Geometry check sheet. Reference: drawing and pictorial views, mm from the part's lowest x, y, z. A direction names the side the tool comes from. Round coordinates to 2 decimals unless told otherwise and drop trailing zeros. Write each loop counter-clockwise with the first axis right and the second up, starting at its lowest first coordinate (ties: lowest second). Pieces come first, ordered by that corner, then holes. Notation, with made-up numbers: M 13.25,54 L 64.25,54 A6 ccw 64.25,59 Z; hole C -18,-22.5 d11. An arc over 180 degrees is marked long. Answer in a Markdown table with one row per item.
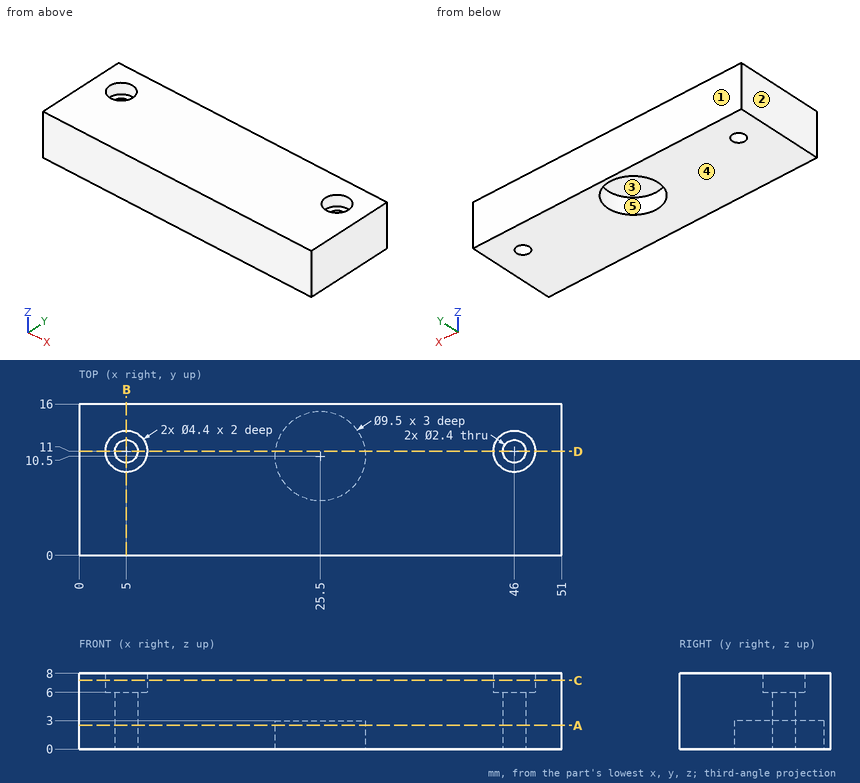
1. Section check A-A, the plane z = 2.5. Record the cut outline in (x, y), and give its area (3 significant figures).
Found:
| item | result |
|---|---|
| outline | M 0,0 L 51,0 L 51,16 L 0,16 Z; hole C 5,11 d2.4; hole C 25.5,10.5 d9.5; hole C 46,11 d2.4 |
| area | 736 mm2 |
2. Scan lines: L1, parallel to X at y = 11, z = 4.25; L2, parallel to Y at x = 46, z = 3.05; L3, parallel to X at y = 11, z = 7.35. Record each from-to range of solid material in increasing order.
Found:
| item | result |
|---|---|
| L1 | x = 0 to 3.8, 6.2 to 44.8, 47.2 to 51 |
| L2 | y = 0 to 9.8, 12.2 to 16 |
| L3 | x = 0 to 2.8, 7.2 to 43.8, 48.2 to 51 |
3. Access from +Z, -Z, +X, -X, +Y, -Y to the whole of each face (thin tool, end or side, straight path). Record for the marked faces 4 and 5.
Found:
| item | result |
|---|---|
| face 4 | -Z, +X, -X, +Y, -Y |
| face 5 | -Z |
4. Section check C-C, the plane z = 7.25. Record the cut outline in (x, y), and give its area (3 significant figures).
Found:
| item | result |
|---|---|
| outline | M 0,0 L 51,0 L 51,16 L 0,16 Z; hole C 5,11 d4.4; hole C 46,11 d4.4 |
| area | 786 mm2 |
5. Section check B-B, the plane x = 5. Record the cut outline in (y, z), and give its area (3 significant figures).
Found:
| item | result |
|---|---|
| outline | M 0,0 L 9.8,0 L 9.8,6 L 8.8,6 L 8.8,8 L 0,8 Z; M 12.2,0 L 16,0 L 16,8 L 13.2,8 L 13.2,6 L 12.2,6 Z |
| area | 105 mm2 |
6. Draft check along X on the marked faces 1, 2 and 3. Enter one of: +X half, -X half, draft (parallel to the pull), parting line (faces both ways), or undercut.
Found:
| item | result |
|---|---|
| face 1 | draft |
| face 2 | -X half |
| face 3 | undercut |
7. Section check D-D, the plane y = 11. Record the cut outline in (x, z), and give its area (3 significant figures).
Found:
| item | result |
|---|---|
| outline | M 0,0 L 3.8,0 L 3.8,6 L 2.8,6 L 2.8,8 L 0,8 Z; M 6.2,0 L 20.78,0 L 20.78,3 L 30.22,3 L 30.22,0 L 44.8,0 L 44.8,6 L 43.8,6 L 43.8,8 L 7.2,8 L 7.2,6 L 6.2,6 Z; M 47.2,0 L 51,0 L 51,8 L 48.2,8 L 48.2,6 L 47.2,6 Z |
| area | 333 mm2 |
8. Go/stop test with flat-tipped pins: pin 1 (4 mm diameter, centred on x = 5, y = 11, fed in from +Z); pin 2 (5 mm diameter, centred on x = 24.5, y = 10.5, fed in from -Z). Record where each tip stops, or that it passes through.
Found:
| item | result |
|---|---|
| pin 1 | stops at z = 6 |
| pin 2 | stops at z = 3 |
